from build123d import *

# Parameters (mm, degrees)
PAD_DEPTH    = 13
SKETCH_R     = 1.565
PAD001_DEPTH = 9
SKETCH001_R  = 6.5
PAD002_DEPTH = 4.5
SKETCH002_R  = 19
PAD003_DEPTH = 65
SKETCH003_R  = 1.5
POCKET_DEPTH = 10


with BuildPart() as part:
    # InvoluteGear → Pad (new body)
    with BuildSketch(Plane.XY):
        with BuildLine():
            Line((3.318799, -0.576475), (3.808072, -0.660799))
            add(Edge.make_bspline(
                [(3.808072, -0.660799), (3.862649, -0.664033), (4.081437, -0.669431), (4.470105, -0.567144), (4.914097, -0.239417)],
                knots=[0, 0, 0, 0, 0, 1, 1, 1, 1, 1], degree=4))
            ThreePointArc((4.914097, -0.239417), (4.919926, 0), (4.914097, 0.239417))
            add(Edge.make_bspline(
                [(4.914097, 0.239417), (4.470105, 0.567144), (4.081437, 0.669431), (3.862649, 0.664033), (3.808072, 0.660799)],
                knots=[0, 0, 0, 0, 0, 1, 1, 1, 1, 1], degree=4))
            Line((3.808072, 0.660799), (3.318799, 0.576475))
            ThreePointArc((3.318799, 0.576475), (3.101267, 0.619895), (2.969549, 0.798377))
            ThreePointArc((2.969549, 0.798377), (2.924499, 0.950227), (2.871689, 1.099557))
            ThreePointArc((2.871689, 1.099557), (2.873343, 1.321373), (3.023808, 1.484363))
            Line((3.023808, 1.484363), (3.469203, 1.703731))
            add(Edge.make_bspline(
                [(3.469203, 1.703731), (3.515258, 1.733194), (3.695434, 1.857427), (3.94975, 2.168633), (4.116314, 2.694741)],
                knots=[0, 0, 0, 0, 0, 1, 1, 1, 1, 1], degree=4))
            ThreePointArc((4.116314, 2.694741), (3.980304, 2.89186), (3.834862, 3.082127))
            add(Edge.make_bspline(
                [(3.834862, 3.082127), (3.283032, 3.086291), (2.90847, 2.94059), (2.73464, 2.807622), (2.692387, 2.772926)],
                knots=[0, 0, 0, 0, 0, 1, 1, 1, 1, 1], degree=4))
            Line((2.692387, 2.772926), (2.346121, 2.417119))
            ThreePointArc((2.346121, 2.417119), (2.144613, 2.324385), (1.933141, 2.391357))
            ThreePointArc((1.933141, 2.391357), (1.80744, 2.487727), (1.676942, 2.577497))
            ThreePointArc((1.676942, 2.577497), (1.5479, 2.757922), (1.573826, 2.978225))
            Line((1.573826, 2.978225), (1.805216, 3.417494))
            add(Edge.make_bspline(
                [(1.805216, 3.417494), (1.825157, 3.4684), (1.897901, 3.674812), (1.920725, 4.076066), (1.746239, 4.5996)],
                knots=[0, 0, 0, 0, 0, 1, 1, 1, 1, 1], degree=4))
            ThreePointArc((1.746239, 4.5996), (1.520341, 4.679127), (1.29084, 4.747568))
            add(Edge.make_bspline(
                [(1.29084, 4.747568), (0.841952, 4.42658), (0.624566, 4.088543), (0.562092, 3.878795), (0.548302, 3.82589)],
                knots=[0, 0, 0, 0, 0, 1, 1, 1, 1, 1], degree=4))
            Line((0.548302, 3.82589), (0.477305, 3.334506))
            ThreePointArc((0.477305, 3.334506), (0.368789, 3.141038), (0.15834, 3.070921))
            ThreePointArc((0.15834, 3.070921), (0, 3.075), (-0.15834, 3.070921))
            ThreePointArc((-0.15834, 3.070921), (-0.368789, 3.141038), (-0.477305, 3.334506))
            Line((-0.477305, 3.334506), (-0.548302, 3.82589))
            add(Edge.make_bspline(
                [(-0.548302, 3.82589), (-0.562092, 3.878795), (-0.624566, 4.088543), (-0.841952, 4.42658), (-1.29084, 4.747568)],
                knots=[0, 0, 0, 0, 0, 1, 1, 1, 1, 1], degree=4))
            ThreePointArc((-1.29084, 4.747568), (-1.520341, 4.679127), (-1.746239, 4.5996))
            add(Edge.make_bspline(
                [(-1.746239, 4.5996), (-1.920725, 4.076066), (-1.897901, 3.674812), (-1.825157, 3.4684), (-1.805216, 3.417494)],
                knots=[0, 0, 0, 0, 0, 1, 1, 1, 1, 1], degree=4))
            Line((-1.805216, 3.417494), (-1.573826, 2.978225))
            ThreePointArc((-1.573826, 2.978225), (-1.5479, 2.757922), (-1.676942, 2.577497))
            ThreePointArc((-1.676942, 2.577497), (-1.80744, 2.487727), (-1.933141, 2.391357))
            ThreePointArc((-1.933141, 2.391357), (-2.144613, 2.324385), (-2.346121, 2.417119))
            Line((-2.346121, 2.417119), (-2.692387, 2.772926))
            add(Edge.make_bspline(
                [(-2.692387, 2.772926), (-2.73464, 2.807622), (-2.90847, 2.94059), (-3.283032, 3.086291), (-3.834862, 3.082127)],
                knots=[0, 0, 0, 0, 0, 1, 1, 1, 1, 1], degree=4))
            ThreePointArc((-3.834862, 3.082127), (-3.980304, 2.89186), (-4.116314, 2.694741))
            add(Edge.make_bspline(
                [(-4.116314, 2.694741), (-3.94975, 2.168633), (-3.695434, 1.857427), (-3.515258, 1.733194), (-3.469203, 1.703731)],
                knots=[0, 0, 0, 0, 0, 1, 1, 1, 1, 1], degree=4))
            Line((-3.469203, 1.703731), (-3.023808, 1.484363))
            ThreePointArc((-3.023808, 1.484363), (-2.873343, 1.321373), (-2.871689, 1.099557))
            ThreePointArc((-2.871689, 1.099557), (-2.924499, 0.950227), (-2.969549, 0.798377))
            ThreePointArc((-2.969549, 0.798377), (-3.101267, 0.619895), (-3.318799, 0.576475))
            Line((-3.318799, 0.576475), (-3.808072, 0.660799))
            add(Edge.make_bspline(
                [(-3.808072, 0.660799), (-3.862649, 0.664033), (-4.081437, 0.669431), (-4.470105, 0.567144), (-4.914097, 0.239417)],
                knots=[0, 0, 0, 0, 0, 1, 1, 1, 1, 1], degree=4))
            ThreePointArc((-4.914097, 0.239417), (-4.919926, 0), (-4.914097, -0.239417))
            add(Edge.make_bspline(
                [(-4.914097, -0.239417), (-4.470105, -0.567144), (-4.081437, -0.669431), (-3.862649, -0.664033), (-3.808072, -0.660799)],
                knots=[0, 0, 0, 0, 0, 1, 1, 1, 1, 1], degree=4))
            Line((-3.808072, -0.660799), (-3.318799, -0.576475))
            ThreePointArc((-3.318799, -0.576475), (-3.101267, -0.619895), (-2.969549, -0.798377))
            ThreePointArc((-2.969549, -0.798377), (-2.924499, -0.950227), (-2.871689, -1.099557))
            ThreePointArc((-2.871689, -1.099557), (-2.873343, -1.321373), (-3.023808, -1.484363))
            Line((-3.023808, -1.484363), (-3.469203, -1.703731))
            add(Edge.make_bspline(
                [(-3.469203, -1.703731), (-3.515258, -1.733194), (-3.695434, -1.857427), (-3.94975, -2.168633), (-4.116314, -2.694741)],
                knots=[0, 0, 0, 0, 0, 1, 1, 1, 1, 1], degree=4))
            ThreePointArc((-4.116314, -2.694741), (-3.980304, -2.89186), (-3.834862, -3.082127))
            add(Edge.make_bspline(
                [(-3.834862, -3.082127), (-3.283032, -3.086291), (-2.90847, -2.94059), (-2.73464, -2.807622), (-2.692387, -2.772926)],
                knots=[0, 0, 0, 0, 0, 1, 1, 1, 1, 1], degree=4))
            Line((-2.692387, -2.772926), (-2.346121, -2.417119))
            ThreePointArc((-2.346121, -2.417119), (-2.144613, -2.324385), (-1.933141, -2.391357))
            ThreePointArc((-1.933141, -2.391357), (-1.80744, -2.487727), (-1.676942, -2.577497))
            ThreePointArc((-1.676942, -2.577497), (-1.5479, -2.757922), (-1.573826, -2.978225))
            Line((-1.573826, -2.978225), (-1.805216, -3.417494))
            add(Edge.make_bspline(
                [(-1.805216, -3.417494), (-1.825157, -3.4684), (-1.897901, -3.674812), (-1.920725, -4.076066), (-1.746239, -4.5996)],
                knots=[0, 0, 0, 0, 0, 1, 1, 1, 1, 1], degree=4))
            ThreePointArc((-1.746239, -4.5996), (-1.520341, -4.679127), (-1.29084, -4.747568))
            add(Edge.make_bspline(
                [(-1.29084, -4.747568), (-0.841952, -4.42658), (-0.624566, -4.088543), (-0.562092, -3.878795), (-0.548302, -3.82589)],
                knots=[0, 0, 0, 0, 0, 1, 1, 1, 1, 1], degree=4))
            Line((-0.548302, -3.82589), (-0.477305, -3.334506))
            ThreePointArc((-0.477305, -3.334506), (-0.368789, -3.141038), (-0.15834, -3.070921))
            ThreePointArc((-0.15834, -3.070921), (0, -3.075), (0.15834, -3.070921))
            ThreePointArc((0.15834, -3.070921), (0.368789, -3.141038), (0.477305, -3.334506))
            Line((0.477305, -3.334506), (0.548302, -3.82589))
            add(Edge.make_bspline(
                [(0.548302, -3.82589), (0.562092, -3.878795), (0.624566, -4.088543), (0.841952, -4.42658), (1.29084, -4.747568)],
                knots=[0, 0, 0, 0, 0, 1, 1, 1, 1, 1], degree=4))
            ThreePointArc((1.29084, -4.747568), (1.520341, -4.679127), (1.746239, -4.5996))
            add(Edge.make_bspline(
                [(1.746239, -4.5996), (1.920725, -4.076066), (1.897901, -3.674812), (1.825157, -3.4684), (1.805216, -3.417494)],
                knots=[0, 0, 0, 0, 0, 1, 1, 1, 1, 1], degree=4))
            Line((1.805216, -3.417494), (1.573826, -2.978225))
            ThreePointArc((1.573826, -2.978225), (1.5479, -2.757922), (1.676942, -2.577497))
            ThreePointArc((1.676942, -2.577497), (1.80744, -2.487727), (1.933141, -2.391357))
            ThreePointArc((1.933141, -2.391357), (2.144613, -2.324385), (2.346121, -2.417119))
            Line((2.346121, -2.417119), (2.692387, -2.772926))
            add(Edge.make_bspline(
                [(2.692387, -2.772926), (2.73464, -2.807622), (2.90847, -2.94059), (3.283032, -3.086291), (3.834862, -3.082127)],
                knots=[0, 0, 0, 0, 0, 1, 1, 1, 1, 1], degree=4))
            ThreePointArc((3.834862, -3.082127), (3.980304, -2.89186), (4.116314, -2.694741))
            add(Edge.make_bspline(
                [(4.116314, -2.694741), (3.94975, -2.168633), (3.695434, -1.857427), (3.515258, -1.733194), (3.469203, -1.703731)],
                knots=[0, 0, 0, 0, 0, 1, 1, 1, 1, 1], degree=4))
            Line((3.469203, -1.703731), (3.023808, -1.484363))
            ThreePointArc((3.023808, -1.484363), (2.873343, -1.321373), (2.871689, -1.099557))
            ThreePointArc((2.871689, -1.099557), (2.924499, -0.950227), (2.969549, -0.798377))
            ThreePointArc((2.969549, -0.798377), (3.101267, -0.619895), (3.318799, -0.576475))
        make_face()
    extrude(amount=PAD_DEPTH)

    # Sketch (on Face81 of Pad) → Pad001 (join)
    with BuildSketch(Plane(origin=(0, 0, 0), x_dir=(1, 0, 0), z_dir=(0, 0, -1))):
        Circle(SKETCH_R)
    extrude(amount=PAD001_DEPTH)

    # Sketch001 (on Face84 of Pad001) → Pad002 (join)
    with BuildSketch(Plane(origin=(0, 0, -9), x_dir=(1, 0, 0), z_dir=(0, 0, -1))):
        Circle(SKETCH001_R)
    extrude(amount=PAD002_DEPTH)

    # Sketch002 (on Face86 of Pad002) → Pad003 (join)
    with BuildSketch(Plane(origin=(0, 0, -13.5), x_dir=(1, 0, 0), z_dir=(0, 0, -1))):
        Circle(SKETCH002_R)
    extrude(amount=PAD003_DEPTH)

    # Sketch003 (on Face86 of Pad003) → Pocket (cut)
    with BuildSketch(Plane.XY.offset(-13.5)):
        with Locations((12.5, 0)):
            Circle(SKETCH003_R)
        with Locations((-12.5, 0)):
            Circle(SKETCH003_R)
    extrude(amount=-POCKET_DEPTH, mode=Mode.SUBTRACT)


solid = part.part
Verification items for the finished model (mm, model axes). A direction names the side the tool comes from. Round coordinates to 2 decimals unless told otherwise and drop trailing zeros. Order: outer loops, then holes, each group sorted by start corner. A loop starts at its lowest first (then second) coordinate and runs counter-clockwise, first axis right, second up. Notation, with made-up numbers: (23, 63) -> (30, 63) arc R9 cw to (30, 77) -> close; hole circle Ø6 at (68.25, 25.25). An arc over 180 degrees is marked (long way). Put each result on its own line as item: value.
1) Depth check by flat-ended pin: pin 1 (1.8 mm diameter, centred on x = -12.5, y = 0, fed in from +Z); pin 2 (8 mm diameter, centred on y = 12, z = -53, fed in from -X); pin 3 (12 mm diameter, centred on y = -9, z = -48, fed in from -X). Enter the tip coordinate at first touch or a pass-through.
Final values:
pin 1: stops at z = -23.5
pin 2: stops at x = -17.23
pin 3: stops at x = -18.76
2) Section check C-C (y = -11). Record the cut outline in (x, z), then the cut area to 3 significant figures.
Final values:
outline: (-15.49, -78.5) -> (15.49, -78.5) -> (15.49, -13.5) -> (-15.49, -13.5) -> close
area: 2,010 mm^2
3) Material ranges on line 1 (Z direction, x = -8.5, y = 4); line 2 (Z direction, x = -2, y = 2); line 3 (Y direction, x = -12, z = -20), recorded low to high.
Final values:
line 1: z = -78.5 to -13.5
line 2: z = -78.5 to -9, 0 to 13
line 3: y = -14.73 to -1.41, 1.41 to 14.73
4) Mould release check, pull along X, two halves, no side actions. Record for faces 1 (the flat face through (-13, 0, -23.5)), 2 (the flat face through (12, 0, -23.5)), 3 (the cylindrical face through (-1.242, 0.952, -4.437)), 4 (the flat face through (8, 0, -13.5)): +X half, -X half, draft (parallel to the pull), parting line (faces both ways), or undercut.
Final values:
face 1: undercut
face 2: undercut
face 3: parting line
face 4: draft
5) Section check A-A (z = -34). Record the cut outline in (x, y).
Final values:
outline: circle Ø38 at (0, 0)
6) Section check B-B (x = -12.5). Record the cut outline in (y, z).
Final values:
outline: (-14.31, -78.5) -> (14.31, -78.5) -> (14.31, -13.5) -> (1.5, -13.5) -> (1.5, -23.5) -> (-1.5, -23.5) -> (-1.5, -13.5) -> (-14.31, -13.5) -> close
7) Set-up check for faces 5 (the cylindrical face through (-5.158, 3.955, -11.218)), 6 (the cylindrical face through (8.767, 16.856, -45.545)), 7 (the flat face through (0, 2, 0)): record each of +Z, -Z, +X, -X, +Y, -Y from which the full face is reachable in a straight line by a thin tool's end or side.
Final values:
face 5: +Z
face 6: +Z, -Z
face 7: none
8) Section check D-D (x = 16). Record the cut outline in (y, z).
Final values:
outline: (-10.25, -78.5) -> (10.25, -78.5) -> (10.25, -13.5) -> (-10.25, -13.5) -> close
